Could you check a few things on this model? Use its own coordinates, in mm. Face numbers are marked on the shaded views. A direction names the side the tool comes from. Round coordinates to 2 decimals unless told otherwise and drop trailing zeros. Loops run counter-clockwise (first coordinate to the right, second up) from the corner with the lowest first, then second, coordinate; pieces in that order, holes last. Notation, with made-up numbers: (84, 36.5) -> (116, 36.5) arc R17 cw to (116, 47.5) -> close; hole circle Ø1 at (-6, 30). An arc over 180 degrees is marked (long way). One line per item, written item: value.
from build123d import *


with BuildPart() as f1:
    # F0 (on Front) → F1 (revolve)
    with BuildSketch(Plane.XZ):
        Polygon((0, 6.1), (0, 8.1), (-5, 8.1), (-5, 6.1), (-4, 6.1), align=None)
        Polygon((0, 0), (0, 6.1), (-4, 6.1), (-4, 0), (-3, 0), align=None)
        Polygon((0, -0.5), (0, 0), (-3, 0), (-3, -4.5), (-1, -4.5), (-1, -1.5), (-0.25, -0.5), align=None)
    revolve(axis=Axis((0, 0, 3.8), (0, 0, -1)))


solid = f1.part
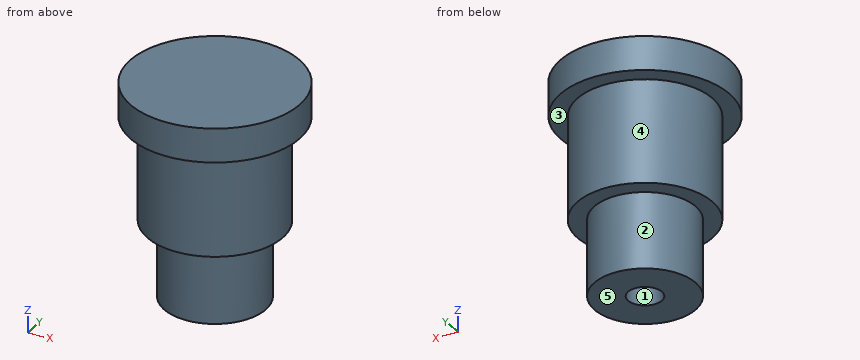
(1) I'm going to push flat-ended pins straight in: pin 1 Ø6 at (x, z) = (0, 0.5) entering from +Y; pin 2 Ø3 at (y, z) = (-0.5, 4.5) entering from -X; pin 3 Ø5 at (y, z) = (-3.5, 2) entering from +X. Where does each tip first touch, or does it pass through?
Recorded:
pin 1: y = 4
pin 2: x = -4
pin 3: x = 3.87
(2) If we section it at D-D, the plane x = 1.25: Please give me the cut outline in (y, z), then the cut area to 3 significant figures.
Recorded:
outline: (-4.84, 6.1) -> (-3.8, 6.1) -> (-3.8, 0) -> (-2.73, 0) -> (-2.73, -4.5) -> (2.73, -4.5) -> (2.73, 0) -> (3.8, 0) -> (3.8, 6.1) -> (4.84, 6.1) -> (4.84, 8.1) -> (-4.84, 8.1) -> close
area: 90.3 mm²
(3) If we section it at A-A, the plane x = 0: Please give me the cut outline in (y, z).
Recorded:
outline: (-5, 6.1) -> (-4, 6.1) -> (-4, 0) -> (-3, 0) -> (-3, -4.5) -> (-1, -4.5) -> (-1, -1.5) -> (-0.25, -0.5) -> (0.25, -0.5) -> (1, -1.5) -> (1, -4.5) -> (3, -4.5) -> (3, 0) -> (4, 0) -> (4, 6.1) -> (5, 6.1) -> (5, 8.1) -> (-5, 8.1) -> close
(4) If I drill on L1, parallel to Z at x = -3, y = 1.75; L2, parallel to Y at x = 0, z = -2.7; L3, parallel to X at y = 0.75, z = -3, over which ranges is the centre line in solid material (lowest first)?
Recorded:
L1: 0 to 8.1
L2: -3 to -1, 1 to 3
L3: -2.9 to -0.66, 0.66 to 2.9
(5) For the marked faces 4 and 5, which set-ups out of +Z, -Z, +X, -X, +Y, -Y let a thin tool reach every point of the face, with its end or its side?
Recorded:
face 4: -Z
face 5: -Z, +X, -X, +Y, -Y
(6) Thinking about a two-plate mould opening in Y: for the marked faces 1, 2 and 3, which applies, released by +Y, released by -Y, zero draft, split by the parting line, or undercut?
Recorded:
face 1: undercut
face 2: split by the parting line
face 3: zero draft
(7) If we section it at C-C, the plane z = 3: Please give me the cut outline in (x, y).
Recorded:
outline: circle Ø8 at (0, 0)
